from build123d import *

# Parameters (mm, degrees)
CYLINDER968_R             = 2.1
CYLINDER968_DEPTH         = 15
CYLINDER969_R             = 2.1
CYLINDER969_DEPTH         = 15
CYLINDER970_R             = 2.1
CYLINDER970_DEPTH         = 15
CYLINDER971_R             = 2.1
CYLINDER971_DEPTH         = 15
FUSION109_PLACEMENT_ANGLE = 90
CYLINDER965_R             = 2
CYLINDER965_DEPTH         = 15
CYLINDER967_R             = 2
CYLINDER967_DEPTH         = 15
CYLINDER966_R             = 2
CYLINDER966_DEPTH         = 15
CYLINDER964_R             = 2
CYLINDER964_DEPTH         = 15
CYLINDER958_R             = 1.25
CYLINDER958_DEPTH         = 15
CYLINDER957_R             = 1.25
CYLINDER957_DEPTH         = 15
CYLINDER956_R             = 1.25
CYLINDER956_DEPTH         = 15
CYLINDER955_R             = 1.25
CYLINDER955_DEPTH         = 15
CYLINDER070_R             = 8.9
CYLINDER070_DEPTH         = 4.2
CYLINDER072_R             = 1.25
CYLINDER072_DEPTH         = 12
BOX005_W                  = 26
BOX005_H                  = 22
BOX005_DEPTH              = 10


with BuildPart() as cylinder968:
    # Cylinder968 → Cylinder968 (new body)
    with BuildSketch(Plane(origin=(7, 0, 0), x_dir=(1, 0, 0), z_dir=(0, 0, 1))):
        Circle(CYLINDER968_R)
    extrude(amount=CYLINDER968_DEPTH)


with BuildPart() as fusion108:
    # Cylinder969 → Cylinder969 (new body)
    with BuildSketch(Plane(origin=(-7, 0, 0), x_dir=(1, 0, 0), z_dir=(0, 0, 1))):
        Circle(CYLINDER969_R)
    extrude(amount=CYLINDER969_DEPTH)

    # Fusion108: union Cylinder968
    add(cylinder968.part)


with BuildPart() as cylinder970:
    # Cylinder970 → Cylinder970 (new body)
    with BuildSketch(Plane(origin=(7, 0, 0), x_dir=(1, 0, 0), z_dir=(0, 0, 1))):
        Circle(CYLINDER970_R)
    extrude(amount=CYLINDER970_DEPTH)


with BuildPart() as fusion110:
    # Cylinder971 → Cylinder971 (new body)
    with BuildSketch(Plane(origin=(-7, 0, 0), x_dir=(1, 0, 0), z_dir=(0, 0, 1))):
        Circle(CYLINDER971_R)
    extrude(amount=CYLINDER971_DEPTH)

    # Fusion109: union Cylinder970
    add(cylinder970.part)


with BuildPart() as fusion110_1:
    # Fusion109 placement: moved
    add(fusion110.part.rotate(Axis((0, 0, 0), (0, 0, 1)), FUSION109_PLACEMENT_ANGLE))

    # Fusion110: union Fusion108
    add(fusion108.part)


with BuildPart() as fusion110_2:
    # Fusion110 placement: moved
    add(fusion110_1.part.moved(Location((0, 0, -14))))


with BuildPart() as cylinder965:
    # Cylinder965 → Cylinder965 (new body)
    with BuildSketch(Plane(origin=(5, 5, -2), x_dir=(1, 0, 0), z_dir=(0, 0, 1))):
        Circle(CYLINDER965_R)
    extrude(amount=CYLINDER965_DEPTH)


with BuildPart() as cylinder967:
    # Cylinder967 → Cylinder967 (new body)
    with BuildSketch(Plane(origin=(5, -5, -2), x_dir=(1, 0, 0), z_dir=(0, 0, 1))):
        Circle(CYLINDER967_R)
    extrude(amount=CYLINDER967_DEPTH)


with BuildPart() as cylinder966:
    # Cylinder966 → Cylinder966 (new body)
    with BuildSketch(Plane(origin=(-5, -5, -2), x_dir=(1, 0, 0), z_dir=(0, 0, 1))):
        Circle(CYLINDER966_R)
    extrude(amount=CYLINDER966_DEPTH)


with BuildPart() as fusion106:
    # Cylinder964 → Cylinder964 (new body)
    with BuildSketch(Plane(origin=(-5, 5, -2), x_dir=(1, 0, 0), z_dir=(0, 0, 1))):
        Circle(CYLINDER964_R)
    extrude(amount=CYLINDER964_DEPTH)

    # Fusion106: union Cylinder965, Cylinder967, Cylinder966
    add(cylinder965.part)
    add(cylinder967.part)
    add(cylinder966.part)


with BuildPart() as cylinder958:
    # Cylinder958 → Cylinder958 (new body)
    with BuildSketch(Plane(origin=(10, -8, -2), x_dir=(1, 0, 0), z_dir=(0, 0, 1))):
        Circle(CYLINDER958_R)
    extrude(amount=CYLINDER958_DEPTH)


with BuildPart() as cylinder957:
    # Cylinder957 → Cylinder957 (new body)
    with BuildSketch(Plane(origin=(10, 8, -2), x_dir=(1, 0, 0), z_dir=(0, 0, 1))):
        Circle(CYLINDER957_R)
    extrude(amount=CYLINDER957_DEPTH)


with BuildPart() as cylinder956:
    # Cylinder956 → Cylinder956 (new body)
    with BuildSketch(Plane(origin=(-10, -8, -2), x_dir=(1, 0, 0), z_dir=(0, 0, 1))):
        Circle(CYLINDER956_R)
    extrude(amount=CYLINDER956_DEPTH)


with BuildPart() as fusion104:
    # Cylinder955 → Cylinder955 (new body)
    with BuildSketch(Plane(origin=(-10, 8, -2), x_dir=(1, 0, 0), z_dir=(0, 0, 1))):
        Circle(CYLINDER955_R)
    extrude(amount=CYLINDER955_DEPTH)

    # Fusion104: union Cylinder958, Cylinder957, Cylinder956
    add(cylinder958.part)
    add(cylinder957.part)
    add(cylinder956.part)


with BuildPart() as cylinder070:
    # Cylinder070 → Cylinder070 (new body)
    with BuildSketch(Plane.XY):
        Circle(CYLINDER070_R)
    extrude(amount=CYLINDER070_DEPTH)


with BuildPart() as fusion036:
    # Cylinder072 → Cylinder072 (new body)
    with BuildSketch(Plane.XY):
        Circle(CYLINDER072_R)
    extrude(amount=CYLINDER072_DEPTH)

    # Fusion036: union Cylinder070
    add(cylinder070.part)


with BuildPart() as diff_lock_planetary_inf_holes:
    # Box005 → Box005 (new body)
    with BuildSketch(Plane(origin=(-13, -11, 0), x_dir=(1, 0, 0), z_dir=(0, 0, 1))):
        with Locations((13, 11)):
            Rectangle(BOX005_W, BOX005_H)
    extrude(amount=BOX005_DEPTH)

    # Cut014011: cut Fusion036
    add(fusion036.part, mode=Mode.SUBTRACT)

    # Cut014048: cut Fusion104
    add(fusion104.part, mode=Mode.SUBTRACT)

    # Cut014053: cut Fusion106
    add(fusion106.part, mode=Mode.SUBTRACT)

    # Cut014054: cut Fusion110
    add(fusion110_2.part, mode=Mode.SUBTRACT)


solid = diff_lock_planetary_inf_holes.part
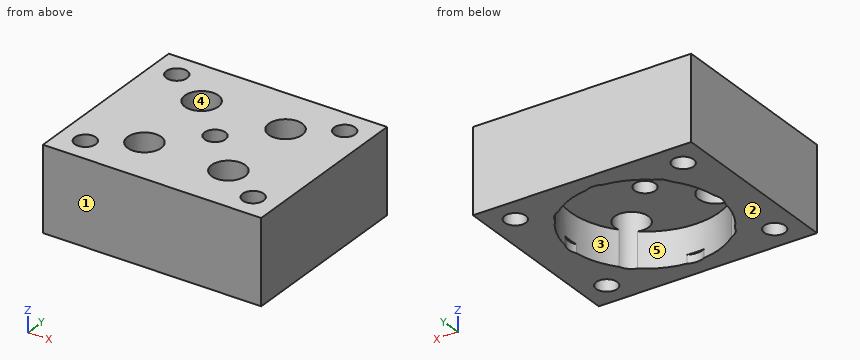
Design review of the part built by this model. Coordinates are the model's own, in mm. Face numbers are marked on the shaded views. A direction names the side the tool comes from. Give positions to 0.01 mm unless a question says otherwise; leave off trailing zeros. Write each loop counter-clockwise with the first axis right and the second up, starting at its lowest first coordinate (ties: lowest second). Pieces come first, ordered by that corner, then holes. Notation, with made-up numbers: M -17.5,7.25 L -3.5,7.25 A15 cw -3.5,35.25 Z; hole C 60.5,15.25 d3. An arc over 180 degrees is marked long. Answer as a JSON object with one key per item and string values. Group by question number.
1) Tool access review of the marked faces 4 and 5: name each direction out of +Z, -Z, +X, -X, +Y, -Y from which nothing blocks a thin tool from reaching the whole face with its end or side.
2) We need section D-D (x = -10). Give the boundary of the cut face in (y, z), and give its area (3 significant figures).
3) Clearance check with a flat-ended pin moving along its axis: pin 1 Ø1 at (x, y) = (4.5, -3) entering from -Z. State where the tip first meets the part, or that it passes through.
4) We need section C-C (y = 0). Give the boundary of the cut face in (x, z).
5) Mouldability with a two-part tool opening along Y and no side actions: class the marked faces 1, 2 and 3 as released by +Y, released by -Y, zero draft, split by the parting line, or undercut.
6) We need section B-B (x = 0). Give the boundary of the cut face in (y, z), and give its area (3 significant figures).
7) We need section A-A (y = 8). Give the boundary of the cut face in (x, z), and give its area (3 significant figures).
8) For line 1 along Y through (x, z) = (-10, 5.75); line 2 along X through (y, z) = (-5, 6); line 3 along Y through (x, z) = (-5, 7), list the stretches that pass through material, from the lowest coordinate up.
Answer key:
{
 "1": {"face 4": "+Z, -Z", "face 5": "-Z"},
 "2": {"outline": "M -11,0 L -9.25,0 L -9.25,10 L -11,10 Z; M -6.75,0 L 6.75,0 L 6.75,10 L -6.75,10 Z; M 9.25,0 L 11,0 L 11,10 L 9.25,10 Z", "area": "170 mm²"},
 "3": {"pin 1": "stops at z = 4.2"},
 "4": {"outline": "M -13,0 L -9.1,0 L -9.1,1 L -8.9,1 L -8.9,4.2 L -1.25,4.2 L -1.25,10 L -13,10 Z; M 1.25,4.2 L 8.9,4.2 L 8.9,1 L 9.1,1 L 9.1,0 L 13,0 L 13,10 L 1.25,10 Z"},
 "5": {"face 1": "released by -Y", "face 2": "zero draft", "face 3": "undercut"},
 "6": {"outline": "M -11,0 L -9.1,0 L -9.1,1 L -8.9,1 L -8.9,4.2 L -1.25,4.2 L -1.25,10 L -11,10 Z; M 1.25,4.2 L 8.9,4.2 L 8.9,1 L 9.1,1 L 9.1,0 L 11,0 L 11,10 L 1.25,10 Z", "area": "130 mm²"},
 "7": {"outline": "M -13,0 L -11.25,0 L -11.25,10 L -13,10 Z; M -8.75,0 L -3.9,0 L -3.9,4.2 L 3.9,4.2 L 3.9,0 L 8.75,0 L 8.75,10 L -8.75,10 Z; M 11.25,0 L 13,0 L 13,10 L 11.25,10 Z", "area": "177 mm²"},
 "8": {"line 1": "y = -11 to -9.25, -6.75 to 6.75, 9.25 to 11", "line 2": "x = -13 to -7, -3 to 3, 7 to 13", "line 3": "y = -11 to -7, -3 to 3, 7 to 11"}
}
